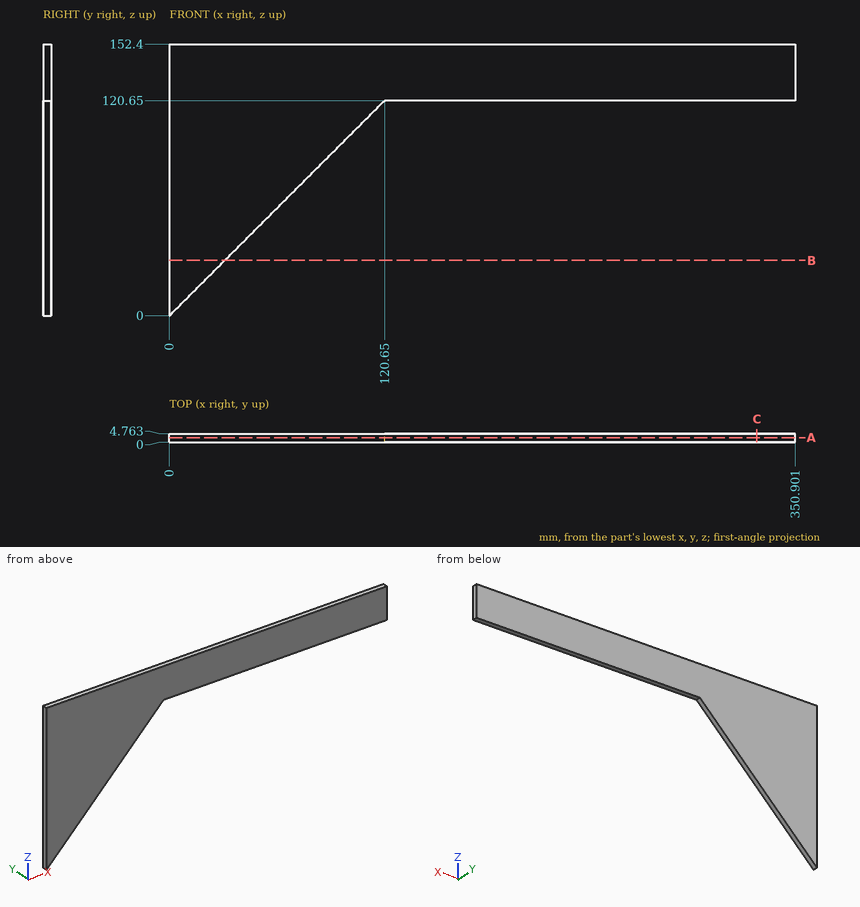
Drawing for the job (mm, zero at the part's lowest x, y, z). Give positions to 0.01 mm unless a question says otherwise; leave off trailing zeros. Loops run counter-clockwise (first coordinate to the right, second up) from the corner with the lowest first, then second, coordinate; pieces in that order, holes last.
(1) Drill centre lines: line 1 along Z through (x, y) = (261, 4.55); line 2 along X through (y, z) = (3.2, 82); line 3 along Z through (x, y) = (95.5, 2.3). Where is each one in solid material? Low to high.
Return value:
line 1: z = 120.65 to 152.4
line 2: x = 0 to 82
line 3: z = 95.5 to 152.4
(2) Band-saw the part on A-A (y = 2.5). Write the cut outline in (x, z), and give its area (3 significant figures).
Return value:
outline: (0, 0) - (120.65, 120.65) - (350.9, 120.65) - (350.9, 152.4) - (0, 152.4) - close
area: 18,400 mm2
(3) Band-saw the part on C-C (x = 329.5). Write the cut outline in (y, z), and give its area (3 significant figures).
Return value:
outline: (0, 120.65) - (4.76, 120.65) - (4.76, 152.4) - (0, 152.4) - close
area: 151 mm2
(4) Pin check, flat tip, straight feed: pin 1 (1 mm diameter, centred on x = 285, y = 2, fed in from -Z). Stop position of the tip, or through.
Return value:
pin 1: stops at z = 120.65
(5) Band-saw the part on B-B (z = 31). Write the cut outline in (x, y), and give its area (3 significant figures).
Return value:
outline: (0, 0) - (31, 0) - (31, 4.76) - (0, 4.76) - close
area: 148 mm2
